Verification items for the finished model (mm, model axes). Give positions to 0.01 mm unless a question says otherwise; leave off trailing zeros. Write each loop counter-clockwise with the first axis right and the second up, starting at its lowest first coordinate (ties: lowest second). Pieces come first, ordered by that corner, then holes. Notation, with made-up numbers: (23, 27.5) - (64, 27.5) arc R16 cw to (64, 31.5) - close; hole circle Ø4 at (12.5, 65.5). An arc over 180 degrees is marked (long way). Answer as a JSON object with one key per item and string values. Group by question number.
Item 1: Scan lines: line 1 along X through (y, z) = (11, 1); line 2 along Y through (x, z) = (10, 1.85); line 3 along Y through (x, z) = (292.5, 1.7). Record each from-to range of solid material in increasing order. Write a range as [from, to].
Item 2: Sectioned sample at B-B, the plane x = 10. Record the boundary of the cut face in (y, z), and give its area (3 significant figures).
Item 3: Sectioned sample at A-A, the plane z = 4.25. Record the boundary of the cut face in (x, y), and give its area (3 significant figures).
Item 4: Sectioned sample at D-D, the plane x = 214. Record the boundary of the cut face in (y, z).
Item 5: Sectioned sample at C-C, the plane y = 12.5. Count the separate pieces of the cut face and the enclosed holes in it, and give its area (3 significant figures).
Item 6: Go/stop test with flat-tipped pins: pin 1 (1 mm diameter, centred on x = 255.5, z = 1.5, fed in from +Y); pin 2 (1 mm diameter, centred on y = -1.5, z = 4.5, fed in from +X); pin 3 (1 mm diameter, centred on x = 82.5, z = 5, fed in from -Y); pin 4 (1.5 mm diameter, centred on x = 172, y = 8.5, fed in from +Z). Record where each tip stops, or that it passes through.
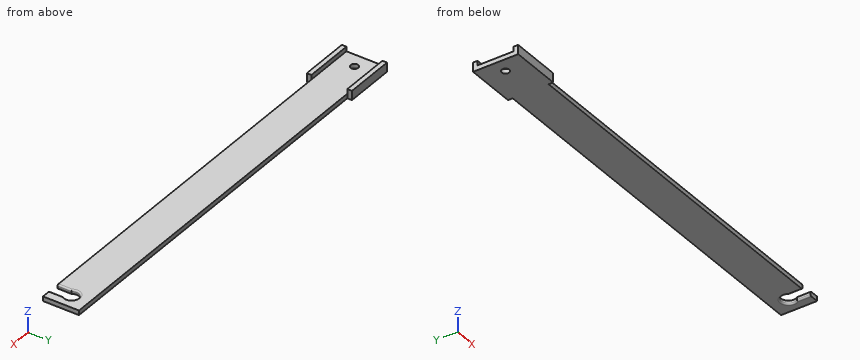
```python
from build123d import *

# Parameters (mm, degrees)
PAD_DEPTH    = 3.2
FILLET_R     = 1
SKETCH001_R  = 2.64391
POCKET_DEPTH = 5
SKETCH002_W  = 35
SKETCH002_H  = 6.4
PAD001_DEPTH = 3.2
SKETCH003_W  = 35
SKETCH003_H  = 6.4
PAD002_DEPTH = 3.2


with BuildPart() as part:
    # Sketch → Pad (new body)
    with BuildSketch(Plane.XY):
        with BuildLine():
            Line((0, 0), (288.43, 0))
            Line((288.43, 0), (288.43, 9.595676))
            ThreePointArc((296.43, 9.408868), (292.616723, 17.498637), (288.43, 9.595676))
            Line((296.43, 0), (296.43, 9.408868))
            Line((296.43, 0), (303, 0))
            Line((303, 0), (303, 25))
            Line((303, 25), (0, 25))
            Line((0, 25), (0, 0))
        make_face()
    extrude(amount=PAD_DEPTH)

    # Fillet
    fillet_edges = [part.edges().sort_by_distance(p)[0] for p in [
        (296.43, 4.704434, 0),
        (292.616723, 17.498637, 0),
        (288.43, 4.797838, 0),
        (296.43, 4.704434, 3.2),
        (288.43, 4.797838, 3.2),
        (292.616723, 17.498637, 3.2),
    ]]
    fillet(fillet_edges, radius=FILLET_R)

    # Sketch001 (on Face6 of Fillet) → Pocket (cut)
    with BuildSketch(Plane.XY.offset(3.2)):
        with Locations((10, 12.5)):
            Circle(SKETCH001_R)
    extrude(amount=-POCKET_DEPTH, mode=Mode.SUBTRACT)

    # Sketch002 (on Face11 of Pocket) → Pad001 (join)
    with BuildSketch(Plane(origin=(0, 25, 0), x_dir=(-1, 0, 0), z_dir=(0, 1, 0))):
        with Locations((-17.5, 3.2)):
            Rectangle(SKETCH002_W, SKETCH002_H)
    extrude(amount=PAD001_DEPTH)

    # Sketch003 (on Face15 of Pad001) → Pad002 (join)
    with BuildSketch(Plane.XZ):
        with Locations((17.5, 3.2)):
            Rectangle(SKETCH003_W, SKETCH003_H)
    extrude(amount=PAD002_DEPTH)


solid = part.part
```
Geometry check:
{
 "1": {"line 1": "[0, 7.82], [12.18, 287.73], [297.27, 303]", "line 2": "[-3.2, 9.86], [15.14, 28.2]", "line 3": "[17.5, 25]"},
 "2": {"outline": "(-3.2, 0) - (9.86, 0) - (9.86, 3.2) - (0, 3.2) - (0, 6.4) - (-3.2, 6.4) - close; (15.14, 0) - (28.2, 0) - (28.2, 6.4) - (25, 6.4) - (25, 3.2) - (15.14, 3.2) - close", "area": "104 mm^2"},
 "3": {"outline": "(0, -3.2) - (35, -3.2) - (35, 0) - (0, 0) - close; (0, 25) - (35, 25) - (35, 28.2) - (0, 28.2) - close", "area": "224 mm^2"},
 "4": {"outline": "(0, 0) - (25, 0) - (25, 3.2) - (0, 3.2) - close"},
 "5": {"separate pieces": "3", "enclosed holes": "0", "area": "920 mm^2"},
 "6": {"pin 1": "y = 25", "pin 2": "x = 35", "pin 3": "through", "pin 4": "z = 3.2"}
}
